from build123d import *

# Parameters (mm, degrees)
BOSS_EXTRUDE1_DEPTH     = 10.16
CUT_EXTRUDE1_START      = -11.16
SKETCH2_R               = 1.7399
CUT_EXTRUDE1_DEPTH      = 12.16
SKETCH3_R               = 2.667
CUT_EXTRUDE2_DEPTH      = 1
CUT_EXTRUDE2_DEPTH_BACK = 11.16


with BuildPart() as part:
    # Sketch1 → Boss-Extrude1 (new body)
    with BuildSketch(Plane.XY):
        with BuildLine():
            Line((0, 6.35), (88.9, 6.35))
            ThreePointArc((88.9, 6.35), (95.25, 0), (88.9, -6.35))
            Line((88.9, -6.35), (0, -6.35))
            ThreePointArc((0, -6.35), (-6.35, 0), (0, 6.35))
        make_face()
    extrude(amount=BOSS_EXTRUDE1_DEPTH)

    # Sketch2 → Cut-Extrude1 (cut)
    with BuildSketch(Plane.XY.offset(10.16).offset(CUT_EXTRUDE1_START)):
        Circle(SKETCH2_R)
    cut_extrude1 = extrude(amount=CUT_EXTRUDE1_DEPTH, mode=Mode.SUBTRACT)

    # Mirror1: Cut-Extrude1 across plane
    add(cut_extrude1.mirror(Plane(origin=(44.45, 0, 0), x_dir=(0, 0, 1), z_dir=(1, 0, 0))), mode=Mode.SUBTRACT)

    # Sketch3 → Cut-Extrude2 (cut, two sides)
    with BuildSketch(Plane.XY.offset(10.16)) as cut_extrude2_sk:
        with Locations((44.2468, 0)):
            Circle(SKETCH3_R)
    extrude(amount=CUT_EXTRUDE2_DEPTH, mode=Mode.SUBTRACT)
    extrude(cut_extrude2_sk.sketch, amount=-CUT_EXTRUDE2_DEPTH_BACK, mode=Mode.SUBTRACT)


solid = part.part
Read the model definition and answer for the solid it produces. Units are mm, in the model's axes. Coordinates: 2 decimals unless noted, no trailing zeros. Order: outer loops, then holes, each group sorted by start corner. A loop starts at its lowest first (then second) coordinate and runs counter-clockwise, first axis right, second up. Notation, with made-up numbers: (2, 44.25) - (42, 44.25) arc R27 cw to (42, 66.25) - close; hole circle Ø9 at (-13, 46). An arc over 180 degrees is marked (long way). Use one line per item in the form item = value.
(1) Section C-C, the plane y = -4 is taken. Give the vertices of the cut face in (x, z), then the cut area to 3 significant figures.
Computed values:
outline = (-4.93, 0) - (93.83, 0) - (93.83, 10.16) - (-4.93, 10.16) - close
area = 1,000 mm²
(2) Straight lines are drawn through the part: L1, parallel to Y at x = 89, z = 4.5; L2, parallel to X at y = 4, z = 9. For each, find the intervals that lie inside material, in ascending order.
Computed values:
L1 = -6.35 to -1.74, 1.74 to 6.35
L2 = -4.93 to 93.83
(3) For a pull along Y with two mould halves and no side action, classify faces 1 (the face through (45, -6.35, 5)), 2 (the face through (44, 6.35, 5)), 3 (the face through (45, -3, 0)), 4 (the face through (-1.38, -1.06, 5.01)) as pulls with the +Y half, pulls with the -Y half, needs draft (parallel to the pull), parting line crosses it, or undercut.
Computed values:
face_1 = pulls with the -Y half
face_2 = pulls with the +Y half
face_3 = needs draft
face_4 = undercut
(4) Section A-A, the plane y = 0 is taken. Give the vertices of the cut face in (x, z), then the cut area to 3 significant figures.
Computed values:
outline = (-6.35, 0) - (-1.74, 0) - (-1.74, 10.16) - (-6.35, 10.16) - close; (1.74, 0) - (41.58, 0) - (41.58, 10.16) - (1.74, 10.16) - close; (46.91, 0) - (87.16, 0) - (87.16, 10.16) - (46.91, 10.16) - close; (90.64, 0) - (95.25, 0) - (95.25, 10.16) - (90.64, 10.16) - close
area = 907 mm²
(5) Given pin 1 Ø1 at (y, z) = (-2.5, 3) entering from +X, flat-ended and moving along its own axis, determine where the tip first touches the part or whether it passes through.
Computed values:
pin_1 = 94.93
(6) Section B-B, the plane z = 8.25 is taken. Give the vertices of the cut face in (x, y), then the cut area to 3 significant figures.
Computed values:
outline = (0, -6.35) - (88.9, -6.35) arc R6.35 ccw to (88.9, 6.35) - (0, 6.35) arc R6.35 ccw to start; hole circle Ø3.48 at (0, 0); hole circle Ø5.33 at (44.25, 0); hole circle Ø3.48 at (88.9, 0)
area = 1,210 mm²
(7) Section D-D, the plane y = 5 is taken. Give the vertices of the cut face in (x, z), then the cut area to 3 significant figures.
Computed values:
outline = (-3.91, 0) - (92.81, 0) - (92.81, 10.16) - (-3.91, 10.16) - close
area = 983 mm²
